from build123d import *

# Parameters (mm, degrees)
SKETCH1_W                   = 82.6516
SKETCH1_H                   = 25.4
BOSS_EXTRUDE1_DEPTH         = 9.5758
SKETCH8_W                   = 2.902818519
SKETCH8_H                   = 9.580147983
BOSS_EXTRUDE4_DEPTH         = 25.4
SKETCH10_R                  = 12.7
BOSS_EXTRUDE5_DEPTH         = 50.1015
SKETCH12_R                  = 6.985
CUT_EXTRUDE2_DEPTH          = 50.8635
CHAMFER1_SIZE               = 2.54
SKETCH14_W                  = 12.7
SKETCH14_H                  = 25.4
BOSS_EXTRUDE6_DEPTH         = 15.24
CUT_EXTRUDE3_REACH          = 81.551
SKETCH18_W                  = 5.842
SKETCH18_H                  = 11.43
F_1_4_CLEARANCE_HOLE2_D     = 6.7564
F_1_4_CLEARANCE_HOLE2_DEPTH = 20.32
F_1_4_CLEARANCE_HOLE2_TIP   = 2.029827343
CHAMFER2_SIZE               = 10.16
SKETCH2_W                   = 22.86
SKETCH2_H                   = 7.2898
CUT_EXTRUDE1_DEPTH          = 69.64351887
SKETCH23_R                  = 3.683
CUT_EXTRUDE6_DEPTH          = 69.64351887


with BuildPart() as part:
    # Sketch1 → Boss-Extrude1 (new body)
    with BuildSketch(Plane(origin=(0, 0, 0), x_dir=(1, 0, 0), z_dir=(0, 1, 0))):
        Rectangle(SKETCH1_W, SKETCH1_H)
    extrude(amount=BOSS_EXTRUDE1_DEPTH)

    # Sketch8 → Boss-Extrude4 (add, through all)
    with BuildSketch(Plane.XY.offset(12.7)):
        with Locations((-1.45140926, 4.790073991)):
            Rectangle(SKETCH8_W, SKETCH8_H)
    extrude(amount=-BOSS_EXTRUDE4_DEPTH)

    # Sketch10 → Boss-Extrude5 (add)
    with BuildSketch(Plane(origin=(0, 9.5758, 0), x_dir=(1, 0, 0), z_dir=(0, 1, 0))):
        with Locations(Location((0, 0, 0), (0, 0, 270))):
            Circle(SKETCH10_R)
    extrude(amount=BOSS_EXTRUDE5_DEPTH)

    # Sketch12 → Cut-Extrude2 (cut)
    with BuildSketch(Plane(origin=(0, 59.6773, 0), x_dir=(1, 0, 0), z_dir=(0, 1, 0))):
        with Locations(Location((0, 0, 0), (0, 0, 270))):
            Circle(SKETCH12_R)
    extrude(amount=-CUT_EXTRUDE2_DEPTH, mode=Mode.SUBTRACT)

    # Chamfer1
    chamfer1_edges = [part.edges().sort_by_distance(p)[0] for p in [
        (0, 59.6773, -12.7),
    ]]
    chamfer(chamfer1_edges, length=CHAMFER1_SIZE)

    # Sketch14 → Boss-Extrude6 (add)
    with BuildSketch(Plane.XY.offset(-6.985)):
        with Locations((0, 41.790845474)):
            Rectangle(SKETCH14_W, SKETCH14_H)
    extrude(amount=-BOSS_EXTRUDE6_DEPTH)

    # Sketch18 → Cut-Extrude3 (cut, up to next)
    with BuildSketch(Plane(origin=(6.35, 0, 0), x_dir=(0, 0, -1), z_dir=(1, 0, 0)), mode=Mode.PRIVATE) as cut_extrude3_sk1:
        with Locations((16.149395763, 44.965845474)):
            Rectangle(SKETCH18_W, SKETCH18_H)
    cut_extrude3_tool1 = extrude(cut_extrude3_sk1.sketch, amount=-CUT_EXTRUDE3_REACH, mode=Mode.PRIVATE) & part.part
    add(cut_extrude3_tool1.solids().sort_by_distance((6.35, 44.965845, -16.149396))[0], mode=Mode.SUBTRACT)

    # 1/4 Clearance Hole2
    with Locations(Plane(origin=(0, 0, -22.225), x_dir=(-1, 0, 0), z_dir=(0, 0, -1))):
        with Locations((0, 44.965845474)):
            Hole(F_1_4_CLEARANCE_HOLE2_D / 2, depth=F_1_4_CLEARANCE_HOLE2_DEPTH)
            with Locations((0, 0, -(F_1_4_CLEARANCE_HOLE2_DEPTH + F_1_4_CLEARANCE_HOLE2_TIP / 2))):  # 118° drill point
                Cone(0, F_1_4_CLEARANCE_HOLE2_D / 2, F_1_4_CLEARANCE_HOLE2_TIP, mode=Mode.SUBTRACT)

    # Chamfer2
    # the kernel refuses this chamfer: 10.16 mm, written as the material it takes off along each edge
    with BuildSketch(Plane(origin=(32.478299158, 29.090845474, -22.225), x_dir=(0, -0.027495876610586265, 0.9996219169112968), z_dir=(-1, 0, 0))) as chamfer2_piece_1_section:
        Polygon((CHAMFER2_SIZE * 0.999621916911, CHAMFER2_SIZE * 0.0274958766106), (-CHAMFER2_SIZE * 0.0274958766106, CHAMFER2_SIZE * 0.999621916911), (0, 0), align=None)
    chamfer2_piece_1 = extrude(amount=64.956598315, mode=Mode.PRIVATE)
    chamfer2_piece_1 = chamfer2_piece_1 - Plane(origin=(0, 32.444576681, 0), x_dir=(0, 0, 1), z_dir=(0, -1, 0)) * Cylinder(12.7, 171, mode=Mode.PRIVATE)
    add(chamfer2_piece_1, mode=Mode.SUBTRACT)

    # Sketch2 → Cut-Extrude1 (cut, through all)
    with BuildSketch(Plane(origin=(0, 9.5758, 0), x_dir=(1, 0, 0), z_dir=(0, 1, 0))):
        with Locations((29.8958, -0.0381)):
            Rectangle(SKETCH2_W, SKETCH2_H)
    cut_extrude1 = extrude(amount=-CUT_EXTRUDE1_DEPTH, mode=Mode.SUBTRACT)

    # Sketch23 → Cut-Extrude6 (cut, through all)
    with BuildSketch(Plane(origin=(0, 9.5758, 0), x_dir=(1, 0, 0), z_dir=(0, 1, 0))):
        with Locations((18.4658, -0.0381)):
            Circle(SKETCH23_R)
    cut_extrude6 = extrude(amount=-CUT_EXTRUDE6_DEPTH, mode=Mode.SUBTRACT)

    # Mirror1: Cut-Extrude1, Cut-Extrude6 across plane
    add(cut_extrude1.mirror(Plane(origin=(0, 0, 0), x_dir=(0, 0, 1), z_dir=(1, 0, 0))), mode=Mode.SUBTRACT)
    add(cut_extrude6.mirror(Plane(origin=(0, 0, 0), x_dir=(0, 0, 1), z_dir=(1, 0, 0))), mode=Mode.SUBTRACT)


solid = part.part
Input: part model. Units: mm. Frame: model coordinates. A direction names the side the tool comes from. Give positions to 0.01 mm unless a question says otherwise; leave off trailing zeros. Write each loop counter-clockwise with the first axis right and the second up, starting at its lowest first coordinate (ties: lowest second). Pieces come first, ordered by that corner, then holes. Notation, with made-up numbers: M -31.75,66 L 12.25,66 A16 ccw 12.25,96 Z; hole C 15,-39.5 d8. An arc over 180 degrees is marked long. Use one line per item in the form item = value.
1. Ray query, L1, parallel to Z at x = 1.5, y = 40 (3 decimals); L2, parallel to Z at x = 3, y = 47 (3 decimals); L3, parallel to Y at x = 36.5, z = -8.5. Return the intervals inside material, ascending.
Outcome:
L1 = -22.225 to -19.07, -13.228 to -6.822, 6.822 to 12.611
L2 = -22.225 to -19.07, -13.228 to -6.308, 6.308 to 12.341
L3 = 0 to 9.58
2. Cut plane D-D on z = -16.5. Return loops of the section in (x, y).
Outcome:
outline = M -6.35,33.53 L 6.35,33.53 L 6.35,39.25 L -6.35,39.25 Z; M -6.35,50.68 L 6.35,50.68 L 6.35,54.49 L -6.35,54.49 Z
3. Mould query, pull axis Y, two halves, no side actions, for faces 4 (the face through (-0.732, 41.668, -9.621)), 5 (the face through (-0.44, 48.315, -20.626)), 6 (the face through (14.784, 4.855, -0.05)), 7 (the face through (-7, 59.677, -2)). Classes: released by +Y, released by -Y, zero draft, split by the parting line, or undercut.
Outcome:
face_4 = undercut
face_5 = undercut
face_6 = zero draft
face_7 = released by +Y
4. Cut plane B-B on x = 25. Return loops of the section in (y, z).
Outcome:
outline = M 0,-12.7 L 9.58,-12.7 L 9.58,-3.61 L 0,-3.61 Z; M 0,3.68 L 9.58,3.68 L 9.58,12.7 L 0,12.7 Z
5. Reachability of faces 1 (the face through (-30, 5, -3.607)), 2 (the face through (0, 8.814, 0)), 3 (the face through (0, 39.251, -16)) from +Z, -Z, +X, -X, +Y, -Y: full face, straight path, thin tool, end or side. Return the list, or none.
Outcome:
face_1 = -X, +Y, -Y
face_2 = +Y
face_3 = +X, -X
6. First-contact query: P1, Ø8.5, axis at x = 18.47, z = 0.04, coming from the +Y side; P2, Ø3.5, axis at x = 0, z = -16.5, coming from the +Y side; P3, Ø1.5, axis at x = -8.5, y = 53, coming from the +Z side. Flat tips, straight axial feed; report the tip coordinate or a pass-through.
Outcome:
P1 = 9.58
P2 = 54.49
P3 = 10.06
7. Cut plane C-C on y = 52.5. Return loops of the section in (x, z) (3 decimals).
Outcome:
outline = M -6.35,-22.225 L 6.35,-22.225 L 6.35,-10.999 A12.7 ccw long -6.35,-10.999 Z; hole C 0,0 d13.97
8. Cut plane A-A on y = 40.5. Return loops of the section in (x, z) (3 decimals).
Outcome:
outline = M -6.35,-22.225 L 6.35,-22.225 L 6.35,-19.07 L -6.35,-19.07 Z; M -6.35,-13.228 L 6.35,-13.228 L 6.35,-10.999 A12.7 ccw long -6.35,-10.999 Z; hole C 0,0 d13.97
